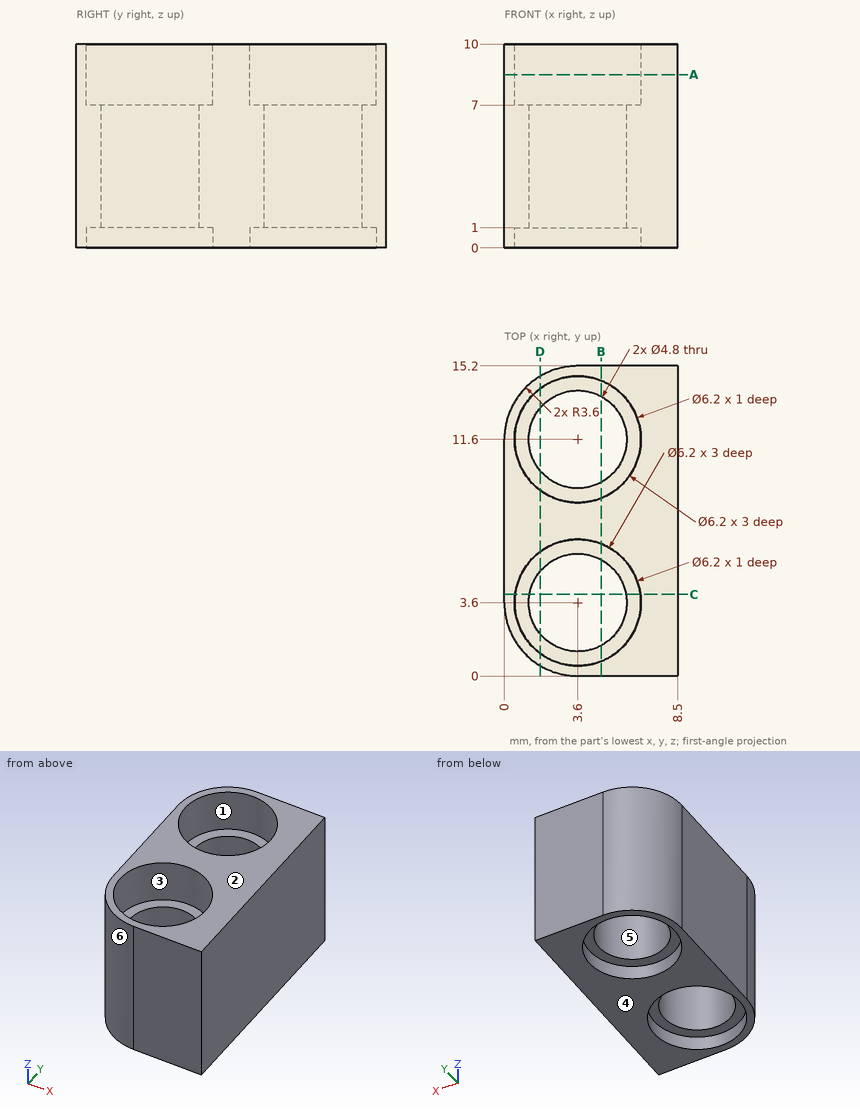
Input: dimensioned drawing with shaded views. Units: mm. Origin: part minimum x, y, z. A direction names the side the tool comes from. Give positions to 0.01 mm unless a question says otherwise; leave off trailing zeros. Loops run counter-clockwise (first coordinate to the right, second up) from the corner with the lowest first, then second, coordinate; pieces in that order, holes last. Notation, with made-up numbers: (-25, 51.25) -> (20, 51.25) arc R11 cw to (20, 70.25) -> close; hole circle Ø1 at (36, -4). An arc over 180 degrees is marked (long way). Use a Markdown table: item, result. Add a question column.
1) First-contact query: pin 1 (3 mm diameter, centred on x = 4.5, y = 4.5, fed in from -Z); pin 2 (5 mm diameter, centred on x = 3.6, y = 11.6, fed in from +Z); pin 3 (2 mm diameter, centred on x = 1.5, z = 8, fed in from +Y). Flat tips, straight axial feed; report the tip coordinate or a pass-through.
2) Pull-direction query (X, two-part tool) for the marked faces 3, 4, 5 and 6; classes: +X half, -X half, draft (parallel to the pull), parting line (faces both ways), or undercut.
3) Reachability of the marked faces 1 and 2 from +Z, -Z, +X, -X, +Y, -Y: full face, straight path, thin tool, end or side. Return the list, or none.
4) Section query A-A, the plane z = 8.5. Return the cut outline in (x, y), then the cut area to 3 significant figures.
5) Section query D-D, the plane x = 1.75. Return the cut outline in (y, z).
6) Section query C-C, the plane y = 4. Return the cut outline in (x, z).
7) Line query: line 1 along Y through (x, z) = (3.6, 9.3); line 2 along Y through (x, z) = (3.6, 5); line 3 along Z through (x, y) = (4.25, 6.25). Output: solid intervals per line, ascending. Write a range as [from, to].
8) Section query B-B, the plane x = 4.75. Return the cut outline in (y, z), then the cut area to 3 significant figures.
Numbers:
| question | item | result |
|---|---|---|
| 1 | pin 1 | stops at z = 1 |
| 1 | pin 2 | stops at z = 7 |
| 1 | pin 3 | stops at y = 15.03 |
| 2 | face 3 | undercut |
| 2 | face 4 | draft |
| 2 | face 5 | undercut |
| 2 | face 6 | -X half |
| 3 | face 1 | +Z |
| 3 | face 2 | +Z, +X, -X, +Y, -Y |
| 4 | outline | (0, 3.6) arc R3.6 ccw to (3.6, 0) -> (8.5, 0) -> (8.5, 15.2) -> (3.6, 15.2) arc R3.6 ccw to (0, 11.6) -> close; hole circle Ø6.2 at (3.6, 3.6); hole circle Ø6.2 at (3.6, 11.6) |
| 4 | area | 63.3 mm2 |
| 5 | outline | (0.51, 0) -> (1.11, 0) -> (1.11, 1) -> (2.07, 1) -> (2.07, 7) -> (1.11, 7) -> (1.11, 10) -> (0.51, 10) -> close; (5.13, 1) -> (6.09, 1) -> (6.09, 0) -> (9.11, 0) -> (9.11, 1) -> (10.07, 1) -> (10.07, 7) -> (9.11, 7) -> (9.11, 10) -> (6.09, 10) -> (6.09, 7) -> (5.13, 7) -> close; (13.13, 1) -> (14.09, 1) -> (14.09, 0) -> (14.69, 0) -> (14.69, 10) -> (14.09, 10) -> (14.09, 7) -> (13.13, 7) -> close |
| 6 | outline | (0, 0) -> (0.53, 0) -> (0.53, 1) -> (1.23, 1) -> (1.23, 7) -> (0.53, 7) -> (0.53, 10) -> (0, 10) -> close; (5.97, 1) -> (6.67, 1) -> (6.67, 0) -> (8.5, 0) -> (8.5, 10) -> (6.67, 10) -> (6.67, 7) -> (5.97, 7) -> close |
| 7 | line 1 | y = [0, 0.5], [6.7, 8.5], [14.7, 15.2] |
| 7 | line 2 | y = [0, 1.2], [6, 9.2], [14, 15.2] |
| 7 | line 3 | z = [1, 7] |
| 8 | outline | (0, 0) -> (0.72, 0) -> (0.72, 1) -> (1.49, 1) -> (1.49, 7) -> (0.72, 7) -> (0.72, 10) -> (0, 10) -> close; (5.71, 1) -> (6.48, 1) -> (6.48, 0) -> (8.72, 0) -> (8.72, 1) -> (9.49, 1) -> (9.49, 7) -> (8.72, 7) -> (8.72, 10) -> (6.48, 10) -> (6.48, 7) -> (5.71, 7) -> close; (13.71, 1) -> (14.48, 1) -> (14.48, 0) -> (15.2, 0) -> (15.2, 10) -> (14.48, 10) -> (14.48, 7) -> (13.71, 7) -> close |
| 8 | area | 55.4 mm2 |
